CAD build for the part. Positions are in the model's coordinates, mm. A direction names the side the tool comes from. Round coordinates to 2 decimals unless told otherwise and drop trailing zeros. Order: outer loops, then holes, each group sorted by start corner. A loop starts at its lowest first (then second) coordinate and runs counter-clockwise, first axis right, second up.
```python
from build123d import *

# Parameters (mm, degrees)
SKETCH1_R                = 15.584715873
SKETCH1_R_2              = 1.25
BOSS_EXTRUDE5_DEPTH      = 6.35
BOSS_EXTRUDE6_START      = -6.35
SKETCH1_7_R              = 15.584715873
SKETCH1_7_R_2            = 1.25
BOSS_EXTRUDE6_DEPTH      = 6.35
BOSS_EXTRUDE7_DEPTH      = 6.35
BOSS_EXTRUDE7_DEPTH_BACK = 25.4


with BuildPart() as part:
    # Sketch1 → Boss-Extrude5 (new body)
    # profile 1 of 3: a face of its own
    with BuildSketch(Plane.XY):
        with BuildLine():
            Line((21.23324901, 27.290268066), (-86.71675099, 27.290268066))
            ThreePointArc((-86.71675099, 27.290268066), (-75.696692713, 22.72561047), (-71.132035117, 11.705552193))
            ThreePointArc((-71.132035117, 11.705552193), (-75.696692713, 0.685493916), (-86.71675099, -3.879163681))
            Line((-86.71675099, -3.879163681), (21.23324901, -3.879163681))
            ThreePointArc((21.23324901, -3.879163681), (5.648533136, 11.705552193), (21.23324901, 27.290268066))
        make_face()
        with BuildLine():
            ThreePointArc((-61.31675099, 7.260552193), (-65.76175099, 11.705552193), (-61.31675099, 16.150552193))
            Line((-61.31675099, 16.150552193), (-4.16675099, 16.150552193))
            ThreePointArc((-4.16675099, 16.150552193), (0.27824901, 11.705552193), (-4.16675099, 7.260552193))
            Line((-4.16675099, 7.260552193), (-61.31675099, 7.260552193))
        make_face(mode=Mode.SUBTRACT)
    # profile 2 of 3: a face of its own
    with BuildSketch(Plane.XY):
        with Locations((-86.71675099, 11.705552193)):
            Circle(SKETCH1_R)
        with Locations((-77.839990601, 16.830552193)):
            Circle(SKETCH1_R_2, mode=Mode.SUBTRACT)
        with Locations((-77.839990601, 6.580552193)):
            Circle(SKETCH1_R_2, mode=Mode.SUBTRACT)
        with Locations((-86.71675099, 1.455552193)):
            Circle(SKETCH1_R_2, mode=Mode.SUBTRACT)
        with Locations((-95.593511379, 6.580552193)):
            Circle(SKETCH1_R_2, mode=Mode.SUBTRACT)
        with Locations((-95.593511379, 16.830552193)):
            Circle(SKETCH1_R_2, mode=Mode.SUBTRACT)
        with Locations((-86.71675099, 21.955552193)):
            Circle(SKETCH1_R_2, mode=Mode.SUBTRACT)
        Polygon((-89.71675099, 9.973501385), (-89.71675099, 13.437603), (-86.71675099, 15.169653808), (-83.71675099, 13.437603), (-83.71675099, 9.973501385), (-86.71675099, 8.241450578), align=None, mode=Mode.SUBTRACT)
    # profile 3 of 3: a face of its own
    with BuildSketch(Plane.XY):
        with BuildLine():
            ThreePointArc((36.817964883, 11.705552193), (32.253307287, 22.72561047), (21.23324901, 27.290268066))
            ThreePointArc((21.23324901, 27.290268066), (5.648533136, 11.705552193), (21.23324901, -3.879163681))
            ThreePointArc((21.23324901, -3.879163681), (32.253307287, 0.685493916), (36.817964883, 11.705552193))
        make_face()
        with Locations((21.23324901, 1.455552193)):
            Circle(SKETCH1_R_2, mode=Mode.SUBTRACT)
        with Locations((12.356488621, 6.580552193)):
            Circle(SKETCH1_R_2, mode=Mode.SUBTRACT)
        with Locations((30.110009399, 6.580552193)):
            Circle(SKETCH1_R_2, mode=Mode.SUBTRACT)
        Polygon((21.23324901, 15.169653808), (24.23324901, 13.437603), (24.23324901, 9.973501385), (21.23324901, 8.241450578), (18.23324901, 9.973501385), (18.23324901, 13.437603), align=None, mode=Mode.SUBTRACT)
        with Locations((12.356488621, 16.830552193)):
            Circle(SKETCH1_R_2, mode=Mode.SUBTRACT)
        with Locations((30.110009399, 16.830552193)):
            Circle(SKETCH1_R_2, mode=Mode.SUBTRACT)
        with Locations((21.23324901, 21.955552193)):
            Circle(SKETCH1_R_2, mode=Mode.SUBTRACT)
    extrude(amount=BOSS_EXTRUDE5_DEPTH)

    # Sketch1<7> → Boss-Extrude6 (add)
    # profile 1 of 2: a face of its own
    with BuildSketch(Plane.XY.offset(BOSS_EXTRUDE6_START)):
        with Locations(Location((-86.71675099, 11.705552193, 0), (0, 0, 90))):
            Circle(SKETCH1_7_R)
        with Locations((-77.839990601, 16.830552193)):
            Circle(SKETCH1_7_R_2, mode=Mode.SUBTRACT)
        with Locations((-77.839990601, 6.580552193)):
            Circle(SKETCH1_7_R_2, mode=Mode.SUBTRACT)
        with Locations((-86.71675099, 1.455552193)):
            Circle(SKETCH1_7_R_2, mode=Mode.SUBTRACT)
        with Locations((-95.593511379, 6.580552193)):
            Circle(SKETCH1_7_R_2, mode=Mode.SUBTRACT)
        with Locations((-95.593511379, 16.830552193)):
            Circle(SKETCH1_7_R_2, mode=Mode.SUBTRACT)
        with Locations((-86.71675099, 21.955552193)):
            Circle(SKETCH1_7_R_2, mode=Mode.SUBTRACT)
        Polygon((-89.71675099, 9.973501385), (-89.71675099, 13.437603), (-86.71675099, 15.169653808), (-83.71675099, 13.437603), (-83.71675099, 9.973501385), (-86.71675099, 8.241450578), align=None, mode=Mode.SUBTRACT)
    # profile 2 of 2: a face of its own
    with BuildSketch(Plane.XY.offset(BOSS_EXTRUDE6_START)):
        with BuildLine():
            ThreePointArc((36.817964883, 11.705552193), (32.253307287, 22.72561047), (21.23324901, 27.290268066))
            ThreePointArc((21.23324901, 27.290268066), (5.648533136, 11.705552193), (21.23324901, -3.879163681))
            ThreePointArc((21.23324901, -3.879163681), (32.253307287, 0.685493916), (36.817964883, 11.705552193))
        make_face()
        with Locations((21.23324901, 1.455552193)):
            Circle(SKETCH1_7_R_2, mode=Mode.SUBTRACT)
        with Locations((12.356488621, 6.580552193)):
            Circle(SKETCH1_7_R_2, mode=Mode.SUBTRACT)
        with Locations((30.110009399, 6.580552193)):
            Circle(SKETCH1_7_R_2, mode=Mode.SUBTRACT)
        Polygon((21.23324901, 15.169653808), (24.23324901, 13.437603), (24.23324901, 9.973501385), (21.23324901, 8.241450578), (18.23324901, 9.973501385), (18.23324901, 13.437603), align=None, mode=Mode.SUBTRACT)
        with Locations((12.356488621, 16.830552193)):
            Circle(SKETCH1_7_R_2, mode=Mode.SUBTRACT)
        with Locations((30.110009399, 16.830552193)):
            Circle(SKETCH1_7_R_2, mode=Mode.SUBTRACT)
        with Locations((21.23324901, 21.955552193)):
            Circle(SKETCH1_7_R_2, mode=Mode.SUBTRACT)
    extrude(amount=BOSS_EXTRUDE6_DEPTH)

    # Sketch1<8> → Boss-Extrude7 (add, two sides: drawn at the far end of the back side and taken through both)
    with BuildSketch(Plane.XY.offset(-BOSS_EXTRUDE7_DEPTH_BACK)):
        Polygon((-86.71675099, 15.169653808), (-83.71675099, 13.437603), (-83.71675099, 9.973501385), (-86.71675099, 8.241450578), (-89.71675099, 9.973501385), (-89.71675099, 13.437603), align=None)
        Polygon((24.23324901, 13.437603), (21.23324901, 15.169653808), (18.23324901, 13.437603), (18.23324901, 9.973501385), (21.23324901, 8.241450578), (24.23324901, 9.973501385), align=None)
    extrude(amount=BOSS_EXTRUDE7_DEPTH + BOSS_EXTRUDE7_DEPTH_BACK)


solid = part.part
```
1. Cut at C-C, the plane z = 3. Give the number of separate pieces and of enclosed holes in the cut face, and give its area (3 significant figures).
2. Cut at A-A, the plane z = -12.5. Write the cut outline in (x, y), and give its area (3 significant figures).
3. Drill centre lines: line 1 (Z direction, x = -63, y = 24.5); line 2 (Y direction, x = 22, z = 2). Where is each one in solid material? Low to high.
4. Cut at D-D, the plane x = -74.5. Write the cut outline in (y, z), and give its area (3 significant figures).
5. Mould opens along Y. For faces 1 (the face through (-85.196, 9.12, -16.008)), 2 (the face through (-85.524, 1.831, -0.089)), 3 (the face through (18.233, 12, -16)), 4 (the face through (28.86, 16.89, -0.09)) say: released by +Y, released by -Y, zero draft, split by the parting line, or undercut.
6. Tool access for faces 5 (the face through (-102.17, 9.68, -1.5)), 6 (the face through (-33, 16.151, 3)), 7 (the face through (-89.717, 12, -16)): list every direction of +Z, -Z, +X, -X, +Y, -Y with a clear straight run to the whole face (end or side of a thin tool).
7. Pin check, flat tips, straight feed: P1, Ø10, axis at x = 11, z = -8.5, coming from the +Y side; P2, Ø1.7, axis at y = 12.5, z = -19, coming from the -X side; P3, Ø2, axis at x = -77.84, y = 16.83, coming from the +Z side; P4, Ø1.5, axis at y = 4, z = -1, coming from the +X side. Stop position of each tip, or through.
8. Cut at B-B, the plane x = -30.5. Write the cut outline in (y, z).
Outcome:
1. separate pieces: 1
1. enclosed holes: 13
1. area: 3,500 mm2
2. outline: (-89.72, 9.97) - (-86.72, 8.24) - (-83.72, 9.97) - (-83.72, 13.44) - (-86.72, 15.17) - (-89.72, 13.44) - close; (18.23, 9.97) - (21.23, 8.24) - (24.23, 9.97) - (24.23, 13.44) - (21.23, 15.17) - (18.23, 13.44) - close
2. area: 62.4 mm2
3. line 1: z = 0 to 6.35
3. line 2: y = -3.86 to 0.47, 2.44 to 20.97, 22.94 to 27.27
4. outline: (-3.88, 0) - (2.03, 0) - (2.03, -6.35) - (21.38, -6.35) - (21.38, 0) - (27.29, 0) - (27.29, 6.35) - (-3.88, 6.35) - close
4. area: 321 mm2
5. face 1: released by -Y
5. face 2: undercut
5. face 3: zero draft
5. face 4: undercut
6. face 5: -Z
6. face 6: +Z, -Z
6. face 7: -Z, -X, +Y, -Y
7. P1: stops at y = 26.2
7. P2: stops at x = -89.72
7. P3: passes through
7. P4: stops at x = 35.18
8. outline: (-3.88, 0) - (7.26, 0) - (7.26, 6.35) - (-3.88, 6.35) - close; (16.15, 0) - (27.29, 0) - (27.29, 6.35) - (16.15, 6.35) - close
